Can you work these out from the model? Positions are in its coordinate system, mm. Face numbers are marked on the shaded views. A direction names the side the tool comes from. Give positions to 0.01 mm unless a question says otherwise; leave off trailing zeros. Write each loop counter-clockwise with the first axis right and the second up, starting at its lowest first coordinate (ties: lowest second). Pieces come first, ordered by that corner, then holes.
1. Suppose I cut it at C-C (x = 12). Please give me the cut outline in (y, z), and give its area (3 significant figures).
2. Suppose I cut it at A-A (z = 0). Please give me the cut outline in (x, y), and give its area (3 significant figures).
3. Suppose I cut it at B-B (z = 11.5). Please give me the cut outline in (x, y), and give its area (3 significant figures).
4. Suppose I cut it at D-D (y = 1.75). Give the number of separate pieces and of enclosed holes in the cut face, and give its area (3 significant figures).
5. If I drill on probe 1 along X at (y, z) = (7.75, -12); probe 2 along Z at (x, y) = (-20, 7.5); probe 3 along Z at (x, y) = (0, 7.75), over which ranges is the centre line in solid material (lowest first)?
6. I'm going to push flat-ended pins straight in: pin 1 (3 mm diameter, centred on x = 20, z = -12, fed in from -Y); pin 2 (2 mm diameter, centred on x = -7.5, y = 10.5, fed in from +Z); pin 3 (1 mm diameter, centred on y = 4, z = -9, fed in from +X); pin 4 (6.5 mm diameter, centred on x = 15.5, y = 9.5, fed in from +Z). Where does each tip first touch, or does it pass through?
7. On a 3-axis mill with a long thin cutter (end or side, diameter ignored), from which of +Z, -Z, +X, -X, +Y, -Y can I reach the whole of each face in a straight line? I mean the marked faces 1, 2 and 3. Say none if no direction works.
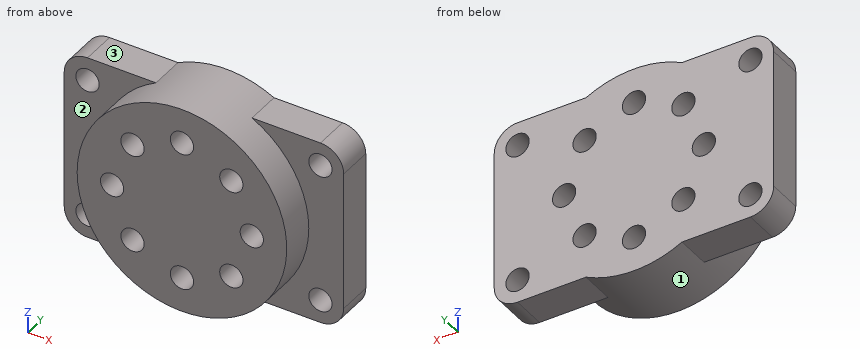
Autodesk Inventor part; units mm, degrees
ref_plane "YZ Plane" through (0, 0, 0) normal (1, 0, 0) x (0, 1, 0)
ref_plane "XZ Plane" through (0, 0, 0) normal (0, 1, 0) x (-1, 0, 0)
ref_plane "XY Plane" through (0, 0, 0) normal (0, 0, 1) x (1, 0, 0)
sketch "Sketch1" plane through (0, 0, 0) normal (0, 1, 0) x (-1, 0, 0)
  circle A0 centre (0, 0) radius 18
  dimension "d0" = 36
extrude "Extrusion1" add sketch "Sketch1" along normal blind 6
sketch "Sketch2" plane through (0, 6, 0) normal (0, 1, 0) x (1, 0, 0)
  circle A0 centre (0, 12) radius 2
  circle A1 centre (-8.4853, 8.4853) radius 2
  circle A2 centre (-12, 0) radius 2
  circle A3 centre (-8.4853, -8.4853) radius 2
  circle A4 centre (0, -12) radius 2
  circle A5 centre (8.4853, -8.4853) radius 2
  circle A6 centre (12, 0) radius 2
  circle A7 centre (8.4853, 8.4853) radius 2
  point P0 (0, 0)
  dimension "d3" = 4
  dimension "d4" = 12
  dimension "d7" = 360
extrude "Extrusion2" cut sketch "Sketch2" against normal through all
sketch "Sketch3" plane through (0, 6, 0) normal (0, 1, 0) x (1, 0, 0)
  line L0 (-24, -16) -> (24, -16)
  line L1 (24, -16) -> (24, 16)
  line L2 (24, 16) -> (-24, 16)
  line L3 (-24, 16) -> (-24, -16)
  line L4 (-24, -16) -> (24, 16) construction
  line L5 (24, -16) -> (-24, 16) construction
  circle A0 centre (20, -12) radius 2
  line L6 (0, 0) -> (0, 16) construction
  line L7 (0, 0) -> (-24, 0) construction
  circle A1 centre (20, 12) radius 2
  circle A2 centre (-20, -12) radius 2
  circle A3 centre (-20, 12) radius 2
  circle A4 centre (0, 0) radius 18
  circle A5 centre (0, -12) radius 2
  circle A6 centre (12, 0) radius 2
  circle A7 centre (-8.4853, 8.4853) radius 2
  circle A8 centre (-8.4853, -8.4853) radius 2
  circle A9 centre (-12, 0) radius 2
  circle A10 centre (0, 12) radius 2
  circle A11 centre (8.4853, -8.4853) radius 2
  circle A12 centre (8.4853, 8.4853) radius 2
  circle A13 centre (0, 0) radius 18
  point P0 (-8.2462, 16)
  point P1 (-8.2462, -16)
  point P2 (8.2462, -16)
  point P3 (8.2462, 16)
  dimension "d11" = 48
  dimension "d12" = 32
  dimension "d13" = 4
  dimension "d14" = 20
  dimension "d15" = 12
extrude "Extrusion3" add sketch "Sketch3" along normal blind 6
fillet "Fillet1" radius 4 4 edges at (24, 9, -16) (24, 9, 16) (-24, 9, -16) (-24, 9, 16)
thread "Thread1"
thread "Thread2"
thread "Thread3"
thread "Thread4"
properties part number "ArmBearingClampingPlate1" material "Aluminum 6061"
Checks:
1. outline: (0, -13.42) - (6, -13.42) - (6, -16) - (12, -16) - (12, -2) - (0, -2) - close; (0, 2) - (12, 2) - (12, 16) - (6, 16) - (6, 13.42) - (0, 13.42) - close
1. area: 305 mm2
2. outline: (-24, 6) - (-18, 6) - (-18, 0) - (-14, 0) - (-14, 12) - (-24, 12) - close; (-10, 0) - (10, 0) - (10, 12) - (-10, 12) - close; (14, 0) - (18, 0) - (18, 6) - (24, 6) - (24, 12) - (14, 12) - close
2. area: 408 mm2
3. outline: (-24, 6) - (-21.94, 6) - (-21.94, 12) - (-24, 12) - close; (-18.06, 6) - (-13.85, 6) - (-13.85, 0) - (-1.94, 0) - (-1.94, 12) - (-18.06, 12) - close; (1.94, 0) - (13.85, 0) - (13.85, 6) - (18.06, 6) - (18.06, 12) - (1.94, 12) - close; (21.94, 6) - (24, 6) - (24, 12) - (21.94, 12) - close
3. area: 361 mm2
4. separate pieces: 1
4. enclosed holes: 8
4. area: 917 mm2
5. probe 1: x = -24 to -22, -18 to -2, 2 to 18, 22 to 24
5. probe 2: z = -16 to -14, -10 to 10, 14 to 16
5. probe 3: z = -18 to -14, -10 to 10, 14 to 18
6. pin 1: passes through
6. pin 2: stops at z = 16.79
6. pin 3: stops at x = 15.87
6. pin 4: stops at z = 16
7. face 1: -Y
7. face 2: -X, -Y
7. face 3: +Z, -X, +Y, -Y
